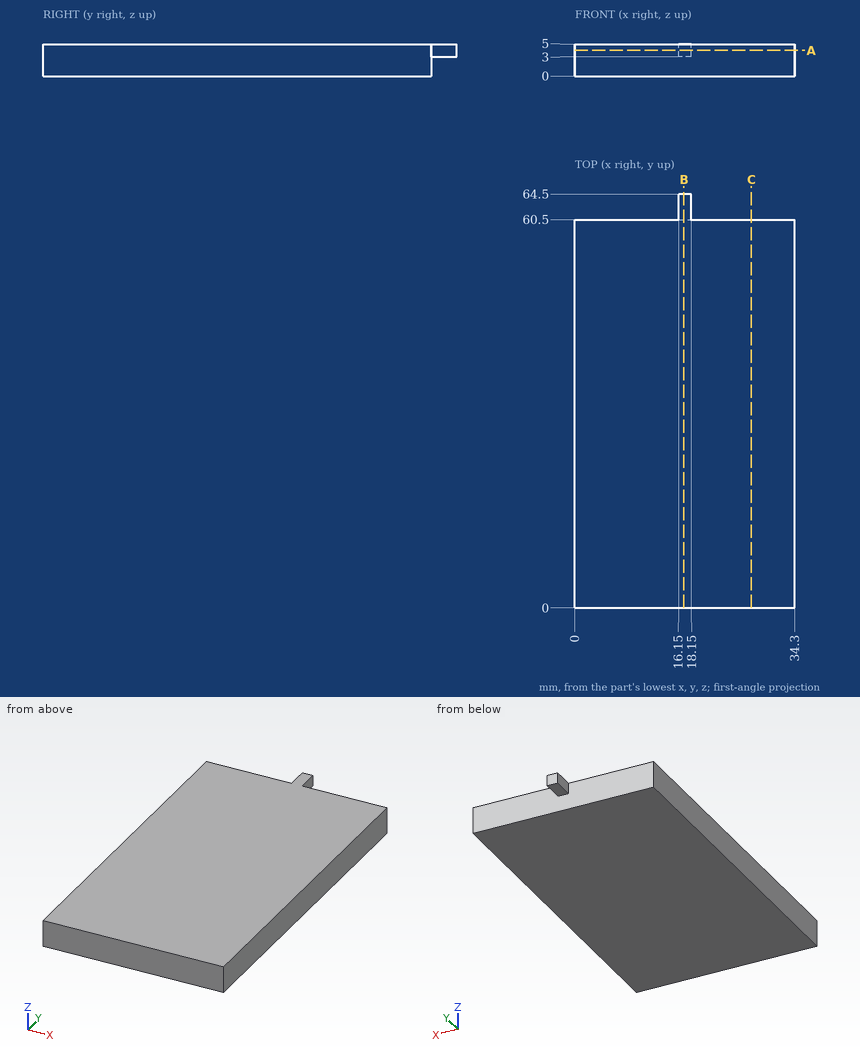
Answer from the drawing. Dimensions are ordinates in mm from the lowest x, y and z of the part. Coordinates: 2 decimals unless noted, no trailing zeros. Loops run counter-clockwise (first coordinate to the right, second up) from the corner with the lowest first, then second, coordinate; pieces in that order, holes last.
Q1. The part is cut by section C-C on x = 27.5. Write down the section's boundary in (y, z), and give its area (4 significant figures).
Q2. Each of these flat-tipped pins is pushed along its axis until it touches: pin 1 Ø2 at (y, z) = (62, 3.5) entering from -X; pin 2 Ø0.6 at (x, y) = (17.5, 62.5) entering from -Z; pin 3 Ø2 at (y, z) = (63.5, 3.5) entering from +X. Where does it stop, or does it pass through?
Q3. The part is cut by section A-A on z = 4. Write down the section's boundary in (x, y), and give its area (3 significant figures).
Q4. The part is cut by section B-B on x = 17. Write down the section's boundary in (y, z).
Q5. Consider probe 1 along Y at (x, z) = (29, 3.3). Determine where the line is inside the solid, lowest interval first.
Results below:
1. outline: (0, 0) - (60.5, 0) - (60.5, 5) - (0, 5) - close
1. area: 302.5 mm2
2. pin 1: stops at x = 16.15
2. pin 2: stops at z = 3
2. pin 3: stops at x = 18.15
3. outline: (0, 0) - (34.3, 0) - (34.3, 60.5) - (18.15, 60.5) - (18.15, 64.5) - (16.15, 64.5) - (16.15, 60.5) - (0, 60.5) - close
3. area: 2,080 mm2
4. outline: (0, 0) - (60.5, 0) - (60.5, 3) - (64.5, 3) - (64.5, 5) - (0, 5) - close
5. probe 1: y = 0 to 60.5
